Check sheet for the modelled part. Datum: model origin and axes. Units: mm. Round coordinates to 2 decimals unless told otherwise and drop trailing zeros. Write each loop counter-clockwise with the first axis right and the second up, starting at its lowest first coordinate (ties: lowest second). Pieces come first, ordered by that corner, then holes.
Item 1: Cross-section at B-B on x = -114. Enter the section's corners in (y, z).
Item 2: Go/stop test with a flat-tipped pin: pin 1 Ø2.5 at (x, y) = (8, 12.07) entering from -Z. Record where the tip stops, or that it passes through.
Item 3: Cross-section at A-A on x = 8. Enter the section's corners in (y, z).
Item 4: Material ranges on line 1 (Y direction, x = -154, z = 19.15); line 2 (Y direction, x = -7, z = 17.6); line 3 (X direction, y = -1, z = 16.3), recorded low to high.
Item 5: Cross-section at C-C on z = 18.7. Count the separate pieces of the cut face and the enclosed holes in it, plus the area to 3 significant figures.
from build123d import *

# Parameters (mm, degrees)
SKETCH_1_W           = 140
SKETCH_1_H           = 40
EXTRUDE_1_DEPTH      = 35
CUT_EXTRUDE_START    = -25
CUT_EXTRUDE_1_DEPTH  = 25
SKETCH_3_W           = 20.946458808
SKETCH_3_H           = 40
CUT_EXTRUDE_2_DEPTH  = 50
SKETCH_4_W           = 119.053541192
SKETCH_4_H           = 40
CUT_EXTRUDE_3_DEPTH  = 16
SKETCH_5_W           = 119.053541192
SKETCH_5_H           = 7.566301572
CUT_EXTRUDE_4_DEPTH  = 33
FILLET_1_R           = 5
SKETCH_6_W           = 119.053541192
SKETCH_6_H           = 32.433698428
EXTRUDE_2_DEPTH      = 3
SKETCH_7_W           = 119.053541192
SKETCH_7_H           = 2.43
CUT_EXTRUDE_5_DEPTH  = 25
FILLET_2_R           = 15
SKETCH_10_W          = 35.667768889
SKETCH_10_H          = 41.429485403
CUT_EXTRUDE_8_DEPTH  = 50
SKETCH_11_W          = 23.137651911
SKETCH_11_H          = 30.003698428
EXTRUDE_3_DEPTH      = 19
SKETCH_12_W          = 18
SKETCH_12_H          = 30.003698428
CUT_EXTRUDE_9_DEPTH  = 150
SKETCH_8_R           = 2
CUT_EXTRUDE_10_DEPTH = 4
SKETCH_13_W          = 4
SKETCH_13_H          = 30.003698428
EXTRUDE_4_DEPTH      = 94
SKETCH_14_R          = 1.6
SKETCH_14_R_2        = 1.75
CUT_EXTRUDE_11_DEPTH = 94
FILLET_4_R           = 10


# Read off the part's stored shape, not the designer's step: 切除-拉伸1
with BuildPart() as part:
    # 草图1 → 凸台-拉伸1 (new body)
    with BuildSketch(Plane.XY):
        Rectangle(SKETCH_1_W, SKETCH_1_H)
    extrude(amount=EXTRUDE_1_DEPTH)

    # 切除-拉伸1 outline → 切除-拉伸1 (cut)
    with BuildSketch(Plane.XY.offset(35).offset(CUT_EXTRUDE_START)):
        with BuildLine():
            ThreePointArc((-65, 0.939701666), (-63.90540849, -0.926084141), (-61.742713718, -0.880933602))
            add(Edge.make_bspline(
                [(-61.742713718, -0.880933602), (-32.663633491, 12.545599653), (-3.21353823, 2.722880029)],
                knots=[0, 0, 0, 1, 1, 1], degree=2))
            add(Edge.make_bspline(
                [(-3.21353823, 2.722880029), (7.778991577, -3.486736981), (19.521763095, -12.075038105), (32.974458778, -10.310789055)],
                knots=[0, 0, 0, 0, 1, 1, 1, 1], degree=3))
            add(Edge.make_bspline(
                [(-1.265226953, 9.621082728), (5.319961167, 7.826511536), (19.072649984, 4.273931772), (30.116773563, 18.680420492), (50.141031873, 7.903163107), (40.152384038, -8.700046956), (32.974458778, -10.310789055)],
                knots=[0, 0, 0, 0, 0.327114299, 0.472643013, 0.672292196, 1, 1, 1, 1], degree=3))
            add(Edge.make_bspline(
                [(-62.225486261, 6.840593766), (-61.950401652, 6.977325912), (-60.645663364, 7.609645854), (-56.787258029, 9.270913685), (-50.206414035, 11.371256832), (-41.494158434, 13.209404155), (-32.600965324, 14.299233241), (-23.90205386, 14.645800276), (-15.41426271, 14.074279585), (-7.837972032, 12.457111584), (-3.215945129, 10.610499943), (-1.265226953, 9.621082728)],
                knots=[0.117371432, 0.117371432, 0.117371432, 0.117371432, 0.12919832, 0.172962492, 0.2758611, 0.378759707, 0.481658315, 0.584556923, 0.687455531, 0.790354139, 0.871867558, 0.871867558, 0.871867558, 0.871867558], degree=3))
            ThreePointArc((-62.225486261, 6.840593766), (-64.250143015, 4.996865242), (-65, 2.363182583))
            Line((-65, 2.363182583), (-65, 0.939701666))
        make_face()
    extrude(amount=CUT_EXTRUDE_1_DEPTH, mode=Mode.SUBTRACT)

    # 草图3 → 切除-拉伸2 (cut)
    with BuildSketch(Plane.XY.offset(35)):
        with Locations((59.526770596, 0)):
            Rectangle(SKETCH_3_W, SKETCH_3_H)
    extrude(amount=-CUT_EXTRUDE_2_DEPTH, mode=Mode.SUBTRACT)

    # 草图4 → 切除-拉伸3 (cut)
    with BuildSketch(Plane(origin=(0, 0, 0), x_dir=(-1, 0, 0), z_dir=(0, 0, -1))):
        with Locations((10.473229404, 0)):
            Rectangle(SKETCH_4_W, SKETCH_4_H)
    extrude(amount=-CUT_EXTRUDE_3_DEPTH, mode=Mode.SUBTRACT)

    # 草图5 → 切除-拉伸4 (cut)
    with BuildSketch(Plane.XY.offset(35)):
        with Locations((-10.473229404, -16.216849214)):
            Rectangle(SKETCH_5_W, SKETCH_5_H)
    extrude(amount=-CUT_EXTRUDE_4_DEPTH, mode=Mode.SUBTRACT)

    # 圆角1
    fillet_1_edges = [part.edges().sort_by_distance(p)[0] for p in [
        (-3.21353823, 2.722880029, 25.5),
        (-1.265226953, 9.621082728, 25.5),
    ]]
    fillet(fillet_1_edges, radius=FILLET_1_R)

    # 草图6 → 凸台-拉伸2 (add)
    with BuildSketch(Plane.XY.offset(35)):
        with Locations((-10.473229404, 3.783150786)):
            Rectangle(SKETCH_6_W, SKETCH_6_H)
    extrude(amount=EXTRUDE_2_DEPTH)

    # 草图7 → 切除-拉伸5 (cut)
    with BuildSketch(Plane(origin=(0, 0, 16), x_dir=(-1, 0, 0), z_dir=(0, 0, -1))):
        with Locations((10.473229404, 18.785)):
            Rectangle(SKETCH_7_W, SKETCH_7_H)
    extrude(amount=-CUT_EXTRUDE_5_DEPTH, mode=Mode.SUBTRACT)

    # 圆角2
    fillet_2_edges = [part.edges().sort_by_distance(p)[0] for p in [
        (49.053541192, 17.57, 27),
        (49.053541192, -12.433698428, 27),
    ]]
    fillet(fillet_2_edges, radius=FILLET_2_R)

    # 草图10 → 切除-拉伸8 (cut)
    with BuildSketch(Plane(origin=(0, 0, 16), x_dir=(-1, 0, 0), z_dir=(0, 0, -1))):
        with Locations((-34.472180194, 2.38587436)):
            Rectangle(SKETCH_10_W, SKETCH_10_H)
    extrude(amount=-CUT_EXTRUDE_8_DEPTH, mode=Mode.SUBTRACT)

    # 草图11 → 凸台-拉伸3 (add)
    with BuildSketch(Plane(origin=(0, 0, 16), x_dir=(-1, 0, 0), z_dir=(0, 0, -1))):
        with Locations((-5.069469793, 2.568150786)):
            Rectangle(SKETCH_11_W, SKETCH_11_H)
    extrude(amount=-EXTRUDE_3_DEPTH)

    # 草图12 → 切除-拉伸9 (cut)
    with BuildSketch(Plane.ZY.offset(70)):
        with Locations((29, 2.568150786)):
            Rectangle(SKETCH_12_W, SKETCH_12_H)
    extrude(amount=-CUT_EXTRUDE_9_DEPTH, mode=Mode.SUBTRACT)

    # 草图8 → 切除-拉伸10 (cut)
    with BuildSketch(Plane(origin=(0, 0, 16), x_dir=(-1, 0, 0), z_dir=(0, 0, -1))):
        with Locations((62, 12.07)):
            Circle(SKETCH_8_R)
        with Locations((-8, 12.07)):
            Circle(SKETCH_8_R)
        with Locations((62, -6.933698428)):
            Circle(SKETCH_8_R)
        with Locations((7, -6.933698428)):
            Circle(SKETCH_8_R)
    extrude(amount=-CUT_EXTRUDE_10_DEPTH, mode=Mode.SUBTRACT)

    # 草图13 → 凸台-拉伸4 (add)
    with BuildSketch(Plane.ZY.offset(70)):
        with Locations((18, 2.568150786)):
            Rectangle(SKETCH_13_W, SKETCH_13_H)
    extrude(amount=EXTRUDE_4_DEPTH)

    # 草图14 → 切除-拉伸11 (cut)
    with BuildSketch(Plane(origin=(0, 0, 16), x_dir=(-1, 0, 0), z_dir=(0, 0, -1))):
        with Locations((154, 2.568150786)):
            Circle(SKETCH_14_R)
        with Locations((114, 12.568150786)):
            Circle(SKETCH_14_R_2)
        with Locations((154, 12.568150786)):
            Circle(SKETCH_14_R_2)
        with Locations((154, -7.431849214)):
            Circle(SKETCH_14_R_2)
        with Locations((114, -7.431849214)):
            Circle(SKETCH_14_R_2)
    extrude(amount=-CUT_EXTRUDE_11_DEPTH, mode=Mode.SUBTRACT)

    # 圆角4
    fillet_4_edges = [part.edges().sort_by_distance(p)[0] for p in [
        (-164, -12.433698428, 18),
        (-164, 17.57, 18),
    ]]
    fillet(fillet_4_edges, radius=FILLET_4_R)


solid = part.part
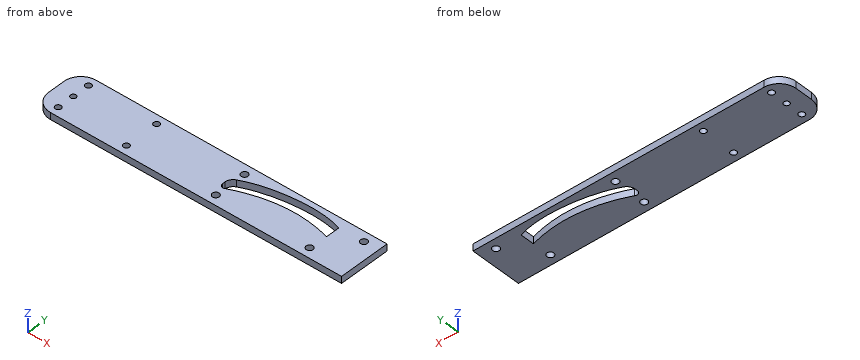
Response values:
1. outline: (-12.43, 16) - (-9.18, 16) - (-9.18, 20) - (-12.43, 20) - close; (-5.68, 16) - (10.82, 16) - (10.82, 20) - (-5.68, 20) - close; (14.32, 16) - (17.57, 16) - (17.57, 20) - (14.32, 20) - close
2. pin 1: passes through
3. outline: (-12.43, 16) - (10.07, 16) - (10.07, 20) - (-12.43, 20) - close; (14.07, 16) - (17.57, 16) - (17.57, 20) - (14.07, 20) - close
4. line 1: y = -12.43 to -9.18, -5.68 to 0.97, 4.17 to 10.82, 14.32 to 17.57
4. line 2: y = -12.43 to -8.93, -4.93 to 3.89, 11.97 to 17.57
4. line 3: x = -164 to -63.76, -61.96 to 16.64
5. separate pieces: 1
5. enclosed holes: 10
5. area: 4,830 mm2
